Build history of the part. All positions in model axes, mm. Face numbers are marked on the shaded views. A direction names the side the tool comes from. Round coordinates to 2 decimals unless told otherwise and drop trailing zeros. Loops run counter-clockwise (first coordinate to the right, second up) from the corner with the lowest first, then second, coordinate; pieces in that order, holes last.
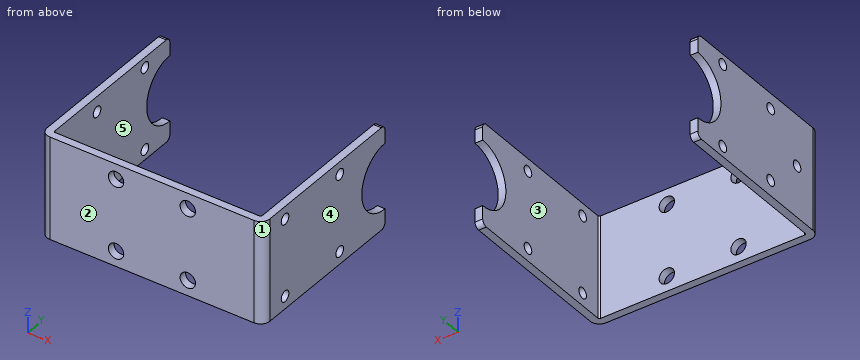
Autodesk Inventor part; units mm, degrees
ref_plane "YZ Plane" through (0, 0, 0) normal (1, 0, 0) x (0, 1, 0)
ref_plane "XZ Plane" through (0, 0, 0) normal (0, 1, 0) x (-1, 0, 0)
ref_plane "XY Plane" through (0, 0, 0) normal (0, 0, 1) x (1, 0, 0)
sketch "Sketch1" plane through (0, 0, 0) normal (0, 1, 0) x (-1, 0, 0)
  line L0 (20.25, -10) -> (-20.25, -10)
  line L1 (-20.25, -10) -> (-20.25, 10)
  line L2 (-20.25, 10) -> (20.25, 10)
  line L3 (20.25, 10) -> (20.25, -10)
  point P0 (0, 0)
  dimension "d0" = 40.5
  dimension "d1" = 20
  dimension "d2" = 10
  dimension "d3" = 20.25
extrude "Plate1" add sketch "Sketch1" along normal blind 1.5
sketch "Sketch2" plane through (21.75, 0, -10) normal (-1, 0, 0) x (0, -1, 0)
  line L0 (0, 20) -> (0, 0)
  line L1 (0, 0) -> (-43.5, 0)
  line L2 (-43.5, 0) -> (-43.5, 20)
  line L3 (-43.5, 20) -> (0, 20)
edge flange "Flange1" height 43.5 angle 90 thickness 1.5 bend radius 0.31 thickness toward (-1, 0, 0) relief tear relief width 1.5 relief depth 0.75 edges at (20.25, 1.5, 0) wall of the first edge with corners at (21.75, 0, 10) (21.75, 0, -10) (21.75, 43.5, -10) (21.75, 43.5, 10)
bend "Bend1"
corner "Corner1"
sketch "Sketch3" plane through (-21.75, 0, 10) normal (1, 0, 0) x (0, 1, 0)
  line L0 (0, -20) -> (0, 0)
  line L1 (0, 0) -> (43.5, 0)
  line L2 (43.5, 0) -> (43.5, -20)
  line L3 (43.5, -20) -> (0, -20)
edge flange "Flange2" height 43.5 angle 90 thickness 1.5 bend radius 0.31 thickness toward (1, 0, 0) relief tear relief width 1.5 relief depth 0.75 edges at (-20.25, 1.5, 0) wall of the first edge with corners at (-21.75, 0, -10) (-21.75, 0, 10) (-21.75, 43.5, 10) (-21.75, 43.5, -10)
bend "Bend2"
corner "Corner2"
sketch "Sketch4" plane through (21.75, 43.5, 10) normal (1, 0, 0) x (0, 0, -1)
  circle A0 centre (10, -9.9) radius 6.4
  line L0 (0, 0) -> (20, 0)
  line L1 (20, 0) -> (20, -41.69)
  point P0 (10, -43.5)
  dimension "d25" = 9.9
  dimension "d26" = 12.8
  dimension "d27" = 10
extrude "Extrusion1" cut sketch "Sketch4" against normal blind 50
sketch "Sketch5" plane through (21.75, 43.5, 10) normal (1, 0, 0) x (0, 0, -1)
  circle A0 centre (10, -9.9) radius 6.4
  line L0 (0, 0) -> (20, 0)
  line L1 (-4, 0) -> (24, 0)
  line L2 (24, 0) -> (24, -9.9)
  line L3 (24, -9.9) -> (-4, -9.9)
  line L4 (-4, -9.9) -> (-4, 0)
  line L5 (0, -41.69) -> (0, 0)
  point P0 (10, -43.5)
  point P1 (20, 0)
  dimension "d30" = 9.9
  dimension "d31" = 28
  dimension "d32" = 4
extrude "Extrusion2" cut sketch "Sketch5" against normal blind 50 contours L3 A0 | A0 L3 L5 L0 L1 L2 | L3 L4 L1 L5 picked at (9.2435, -7.9053)
fillet "Fillet1" radius 1 4 edges at (-21, 33.6, 10) (-21, 33.6, -10) (21, 33.6, -10) (21, 33.6, 10)
sketch "Sketch11" plane through (0, 1.5, 0) normal (0, 1, 0) x (1, 0, 0)
  circle A0 centre (7, 7) radius 1.5
  line L0 (-19.94, 10) -> (19.94, 10)
  line L1 (-19.94, 10) -> (-19.94, -10)
  circle A1 centre (-7, 7) radius 1.5
  circle A2 centre (7, -7) radius 1.5
  circle A3 centre (-7, -7) radius 1.5
  point P0 (0, 0)
  dimension "d71" = 7
  dimension "d72" = 3
  dimension "d73" = 7
  dimension "d76" = 14
  dimension "d79" = 14
extrude "Extrusion3" cut sketch "Sketch11" against normal through all
sketch "Sketch12" plane through (-21.75, 1.81, -10) normal (-1, 0, 0) x (0, 0, 1)
  circle A0 centre (18, 24.89) radius 0.7835
  circle A1 centre (10, 24.79) radius 0.7835
  circle A2 centre (17, 11.67) radius 0.7835
  circle A3 centre (3, 11.67) radius 0.7835
  circle A4 centre (10, 4.37) radius 0.7835
  circle A5 centre (2, 24.89) radius 0.7835
  point P0 (10, -1.81)
hole "Hole6" at (-21.75, 26.7, -8) at (-21.75, 26.7, 8) at (-21.75, 13.48, 7) at (-21.75, 6.18, 0) at (-21.75, 13.48, -7) direction (1, 0, 0) diameter 2.1 depth 1.5
sketch "Sketch13" plane through (21.75, 1.81, 10) normal (1, 0, 0) x (0, 0, -1)
  circle A0 centre (17.525, 4.19) radius 0.7835
  circle A1 centre (2.475, 4.19) radius 0.7835
  circle A2 centre (2.475, 19.29) radius 0.7835
  circle A3 centre (17.525, 19.29) radius 0.7835
  point P0 (10, -1.81)
hole "Hole7" at (21.75, 21.1, 7.525) at (21.75, 21.1, -7.525) at (21.75, 6, -7.525) at (21.75, 6, 7.525) direction (-1, 0, 0) diameter 2.1 depth 1.5
equation "\"d89\" = Thickness"
equation "\"d96\" = Thickness"
equation "\"d4\" = Thickness"
equation "\"d5\" = BendReliefWidth"
equation "\"d6\" = BendReliefDepth"
equation "\"d7\" = MinimumRemnant"
equation "\"d8\" = TransitionRadius"
equation "\"d11\" = BendRadius"
equation "\"d12\" = CornerReliefSize"
equation "\"d13\" = GapSize"
equation "\"d14\" = JacobiRadiusSize"
equation "\"d15\" = BendReliefWidth"
equation "\"d16\" = BendReliefDepth"
equation "\"d17\" = MinimumRemnant"
equation "\"d18\" = TransitionRadius"
equation "\"d21\" = BendRadius"
equation "\"d22\" = CornerReliefSize"
equation "\"d23\" = GapSize"
equation "\"d24\" = JacobiRadiusSize"
equation "\"BendReliefWidth\" = Thickness"
equation "\"BendReliefDepth\" = 0.5 * Thickness"
equation "\"CornerReliefSize\" = 4 * Thickness"
equation "\"MinimumRemnant\" = 2 * Thickness"
equation "\"TransitionRadius\" = BendRadius"
equation "\"JacobiRadiusSize\" = BendRadius"
equation "\"GapSize\" = Thickness"
properties part number "axis_10_top_frame" material "Aluminum 6061-AHC"
(1) Slice it at B-B on y = 18.5. List the corners of the cut face in (x, z), plus the area to 3 significant figures.
Responses:
outline: (-21.75, -10) - (-20.25, -10) - (-20.25, 10) - (-21.75, 10) - close; (20.25, -10) - (21.75, -10) - (21.75, 10) - (20.25, 10) - close
area: 60.0 mm2
(2) Slice it at D-D on x = 2. List the corners of the cut face in (y, z), plus the area to 3 significant figures.
Responses:
outline: (0, -10) - (1.5, -10) - (1.5, 10) - (0, 10) - close
area: 30.0 mm2
(3) Slice it at C-C on y = 26.7. List the corners of the cut face in (x, z).
Responses:
outline: (-21.75, -10) - (-20.25, -10) - (-20.25, -9.05) - (-21.75, -9.05) - close; (-21.75, -6.95) - (-20.25, -6.95) - (-20.25, 6.95) - (-21.75, 6.95) - close; (-21.75, 9.05) - (-20.25, 9.05) - (-20.25, 10) - (-21.75, 10) - close; (20.25, -10) - (21.75, -10) - (21.75, 10) - (20.25, 10) - close
(4) Pull direction X, two halves, no side cores. Call the marked faces 1, 2 and 3: +X half, -X half, draft (parallel to the pull), parting line (faces both ways), or undercut.
Responses:
face 1: +X half
face 2: draft
face 3: undercut
(5) Pin check, flat tips, straight feed: P1, Ø12, axis at x = -15.5, z = 4, coming from the +Y side; P2, Ø8, axis at x = 7, z = -2.5, coming from the +Y side; P3, Ø1.8, axis at x = -7, z = -7, coming from the -Y side; P4, Ø1.7, axis at y = 6, z = 7.525, coming from the +X side. Stop position of each tip, or through.
Responses:
P1: stops at y = 33.6
P2: stops at y = 1.5
P3: passes through
P4: stops at x = -20.25
(6) Slice it at A-A on x = -7. List the corners of the cut face in (y, z), plus the area to 3 significant figures.
Responses:
outline: (0, -10) - (1.5, -10) - (1.5, -8.5) - (0, -8.5) - close; (0, -5.5) - (1.5, -5.5) - (1.5, 5.5) - (0, 5.5) - close; (0, 8.5) - (1.5, 8.5) - (1.5, 10) - (0, 10) - close
area: 21.0 mm2
(7) Probe line 1 (Z direction, x = 20.6, y = 6) (3 decimals); line 2 (Z direction, x = -20.65, y = 13.48); line 3 (X direction, y = 17, z = -8.5). List the from-to ranges inside material, lowest first.
Responses:
line 1: z = -10 to -8.575, -6.475 to 6.475, 8.575 to 10
line 2: z = -10 to -8.05, -5.95 to 5.95, 8.05 to 10
line 3: x = -21.75 to -20.25, 20.25 to 21.75
(8) Which spindle directions (+Z, -Z, +X, -X, +Y, -Y) get a long thin tool onto all of the face, cutting with end or side? Do the marked faces 4 and 5. Say none if no direction does.
Responses:
face 4: +Z, -Z, +X, +Y, -Y
face 5: +Z, -Z, +Y
